Geometry: see drawing. Coordinates: mm, zero at the bounding-box minimum. Round coordinates to 2 decimals unless told otherwise and drop trailing zeros. Loops run counter-clockwise (first coordinate to the right, second up) from the corner with the lowest first, then second, coordinate; pieces in that order, holes last. Notation, with made-up numbers: (9.5, 86) - (59.5, 86) arc R27 cw to (59.5, 119) - close; hole circle Ø2 at (-34.75, 21.25). An arc over 180 degrees is marked (long way). Use CSV: the item, a comma, the result in double quotes. Start each with the question number.
1. Cut plane B-B (x = 63.5). Return loops of the section in (y, z).
2. Cut plane A-A (z = 1.65). Return loops of the section in (x, y) (1 decimal), and give its area (3 significant figures).
3. Pin query (flat end, axial travel): P1, Ø3, axis at x = 45.5, y = 19.5, coming from the -Z side; P2, Ø0.8, axis at x = 30.5, z = 2, coming from the -Y side. Return the tip coordinate at first contact, or that it passes through.
4. Material intervals for probe 1 along Y at (x, z) = (33, 1.6), sorted ascending. Write a range as from..to.
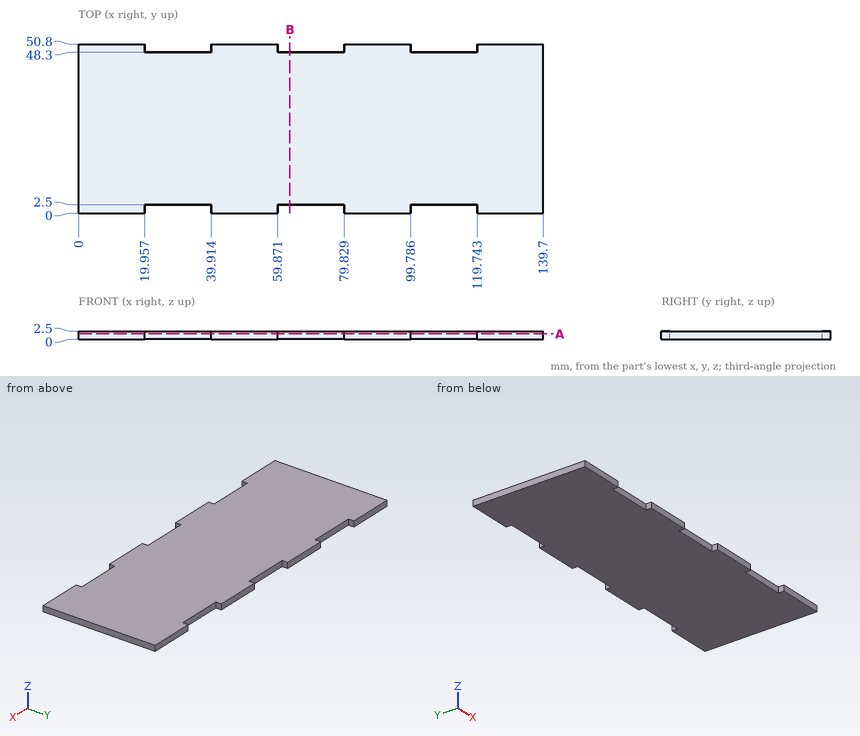
Established:
1,outline,"(2.5, 0) - (48.3, 0) - (48.3, 2.5) - (2.5, 2.5) - close"
2,outline,"(0, 0) - (20, 0) - (20, 2.5) - (39.9, 2.5) - (39.9, 0) - (59.9, 0) - (59.9, 2.5) - (79.8, 2.5) - (79.8, 0) - (99.8, 0) - (99.8, 2.5) - (119.7, 2.5) - (119.7, 0) - (139.7, 0) - (139.7, 50.8) - (119.7, 50.8) - (119.7, 48.3) - (99.8, 48.3) - (99.8, 50.8) - (79.8, 50.8) - (79.8, 48.3) - (59.9, 48.3) - (59.9, 50.8) - (39.9, 50.8) - (39.9, 48.3) - (20, 48.3) - (20, 50.8) - (0, 50.8) - close"
2,area,"6,800 mm2"
3,P1,"stops at z = 0"
3,P2,"stops at y = 2.5"
4,probe 1,"y = 2.5..48.3"
